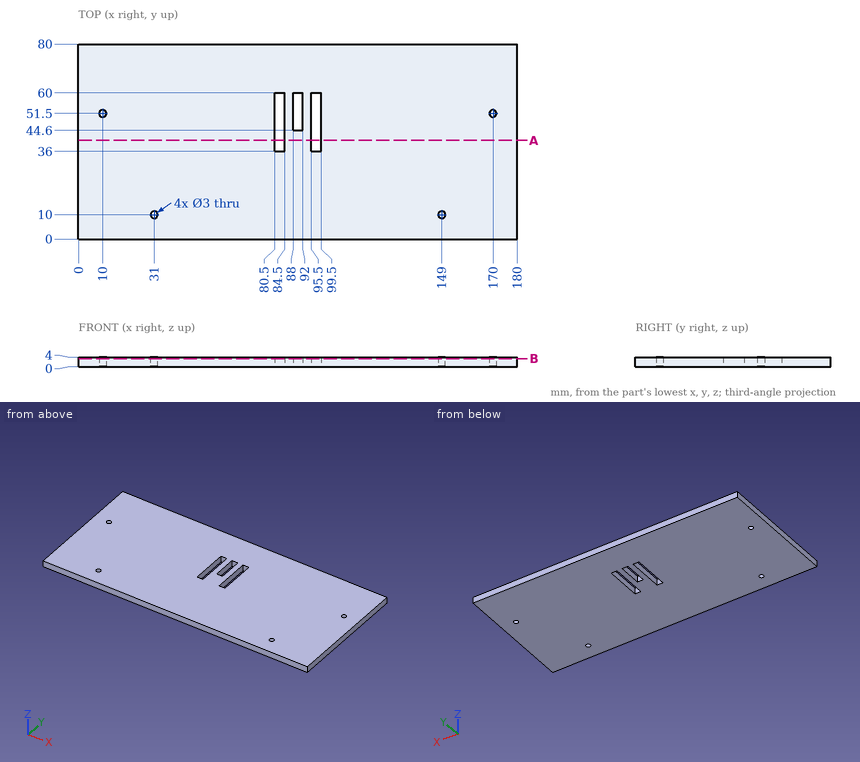
Source: three-view drawing plus pictorial views. Frame: mm from the lowest corner of the part. Coordinates: 2 decimals unless noted, no trailing zeros. Loops run counter-clockwise (first coordinate to the right, second up) from the corner with the lowest first, then second, coordinate; pieces in that order, holes last. Notation, with made-up numbers: (-34, 38) - (2, 38) arc R19 cw to (2, 49) - close; hole circle Ø5 at (8, 59.5). An arc over 180 degrees is marked (long way). One line per question, with ' | ' between items.
1) Section B-B, the plane z = 3.4. Return loops of the section in (x, y), then the cut area to 3 significant figures.
Report:
outline: (0, 0) - (180, 0) - (180, 80) - (0, 80) - close; hole circle Ø3 at (10, 51.5); hole circle Ø3 at (31, 10); hole (80.5, 36) - (84.5, 36) - (84.5, 60) - (80.5, 60) - close; hole (88, 44.6) - (92, 44.6) - (92, 60) - (88, 60) - close; hole (95.5, 36) - (99.5, 36) - (99.5, 60) - (95.5, 60) - close; hole circle Ø3 at (149, 10); hole circle Ø3 at (170, 51.5) | area: 14,100 mm²
2) First-contact query: P1, Ø1.8, axis at x = 170, y = 51.5, coming from the +Z side. Flat tip, straight axial feed; report the tip coordinate or a pass-through.
Report:
P1: passes through
3) Line query: line 1 along X through (y, z) = (44.5, 3.3); line 2 along Y through (x, z) = (149, 1); line 3 along Y through (x, z) = (98.5, 0.7). Output: solid intervals per line, ascending.
Report:
line 1: x = 0 to 80.5, 84.5 to 95.5, 99.5 to 180 | line 2: y = 0 to 8.5, 11.5 to 80 | line 3: y = 0 to 36, 60 to 80
4) Section A-A, the plane y = 40.5. Return loops of the section in (x, z), then the cut area to 3 significant figures.
Report:
outline: (0, 0) - (80.5, 0) - (80.5, 4) - (0, 4) - close; (84.5, 0) - (95.5, 0) - (95.5, 4) - (84.5, 4) - close; (99.5, 0) - (180, 0) - (180, 4) - (99.5, 4) - close | area: 688 mm²
